CAD build for the part. Positions are in the model's coordinates, mm. A direction names the side the tool comes from. Give positions to 0.01 mm unless a question says otherwise; leave off trailing zeros. Loops run counter-clockwise (first coordinate to the right, second up) from the corner with the lowest first, then second, coordinate; pieces in that order, holes last. Notation, with made-up numbers: M 46.5,35.25 L 76.5,35.25 A22 cw 76.5,43.25 Z; hole C 71.5,73.25 d3. An arc over 180 degrees is marked long. Answer as CSV lines item,"result".
from build123d import *

# Parameters (mm, degrees)
F0_W     = 177.8
F0_H     = 177.8
F1_DEPTH = 12.7
F2_W     = 177.8
F2_H     = 177.8
F2_W_2   = 165.1
F2_H_2   = 165.1
F3_DEPTH = 50.8
F4_W     = 76.2
F4_H     = 25.4
F5_DEPTH = 177.8
F6_W     = 76.2
F6_H     = 25.4
F7_DEPTH = 177.8
F8_R     = 1.5875
F9_DEPTH = 25.4


with BuildPart() as f1:
    # F0 (on Top) → F1 (new body)
    with BuildSketch(Plane.XY):
        with Locations((88.9, 88.9)):
            Rectangle(F0_W, F0_H)
    extrude(amount=F1_DEPTH)

    # F2 (on face) → F3 (join)
    with BuildSketch(Plane.XY.offset(12.7)):
        with Locations((88.9, 88.9)):
            Rectangle(F2_W, F2_H)
        with Locations((88.9, 88.9)):
            Rectangle(F2_W_2, F2_H_2, mode=Mode.SUBTRACT)
    extrude(amount=F3_DEPTH)

    # F4 (on face) → F5 (cut, through all)
    with BuildSketch(Plane.YZ.offset(177.8)):
        with Locations((88.9, 38.1)):
            Rectangle(F4_W, F4_H)
    extrude(amount=-F5_DEPTH, mode=Mode.SUBTRACT)

    # F6 (on face) → F7 (cut, through all)
    with BuildSketch(Plane.XZ):
        with Locations((88.9, 38.1)):
            Rectangle(F6_W, F6_H)
    extrude(amount=-F7_DEPTH, mode=Mode.SUBTRACT)

    # F8 (on face) → F9 (join, through all)
    with BuildSketch(Plane.XY.offset(25.4)):
        with Locations((174.625, 69.85)):
            Circle(F8_R)
        with Locations((174.625, 57.15)):
            Circle(F8_R)
        with Locations((174.625, 82.55)):
            Circle(F8_R)
        with Locations((174.625, 107.95)):
            Circle(F8_R)
        with Locations((174.625, 120.65)):
            Circle(F8_R)
        with Locations((174.625, 95.25)):
            Circle(F8_R)
        with Locations((69.85, 174.625)):
            Circle(F8_R)
        with Locations((57.15, 174.625)):
            Circle(F8_R)
        with Locations((82.55, 174.625)):
            Circle(F8_R)
        with Locations((107.95, 174.625)):
            Circle(F8_R)
        with Locations((120.65, 174.625)):
            Circle(F8_R)
        with Locations((95.25, 174.625)):
            Circle(F8_R)
        with Locations((69.85, 3.175)):
            Circle(F8_R)
        with Locations((57.15, 3.175)):
            Circle(F8_R)
        with Locations((82.55, 3.175)):
            Circle(F8_R)
        with Locations((107.95, 3.175)):
            Circle(F8_R)
        with Locations((120.65, 3.175)):
            Circle(F8_R)
        with Locations((95.25, 3.175)):
            Circle(F8_R)
        with Locations((3.175, 69.85)):
            Circle(F8_R)
        with Locations((3.175, 57.15)):
            Circle(F8_R)
        with Locations((3.175, 82.55)):
            Circle(F8_R)
        with Locations((3.175, 107.95)):
            Circle(F8_R)
        with Locations((3.175, 120.65)):
            Circle(F8_R)
        with Locations((3.175, 95.25)):
            Circle(F8_R)
    extrude(amount=F9_DEPTH)


solid = f1.part
1) Which spindle directions (+Z, -Z, +X, -X, +Y, -Y) get a long thin tool onto all of the face, cutting with end or side? Do faces 5 (the face through (175, 127, 38)), 6 (the face through (50.8, 3, 38)), 7 (the face through (171.45, 88, 55)). Say none if no direction does.
Answer below:
face 5,"+X, -X"
face 6,"+Y, -Y"
face 7,"+Z"
2) Band-saw the part on C-C on z = 47. Give the number of separate pieces and of enclosed holes in the cut face, and give its area (3 significant figures).
Answer below:
separate pieces,"28"
enclosed holes,"0"
area,"2,610 mm^2"
3) Band-saw the part on A-A on x = 142.5. Give the cut face in (y, z), and give its area (3 significant figures).
Answer below:
outline,"M 0,0 L 177.8,0 L 177.8,63.5 L 171.45,63.5 L 171.45,12.7 L 6.35,12.7 L 6.35,63.5 L 0,63.5 Z"
area,"2,900 mm^2"
4) Mould opens along Z. For faces 1 (the face through (88, 90, 0)), 2 (the face through (88, 175, 25.4)), 3 (the face through (88, 6.35, 55)), 4 (the face through (88, 175, 50.8)) say: +Z half, -Z half, draft (parallel to the pull), parting line (faces both ways), or undercut.
Answer below:
face 1,"-Z half"
face 2,"undercut"
face 3,"draft"
face 4,"undercut"
5) Flat gauge pins, fed straight in: pin 1 (15 mm diameter, centred on y = 109, z = 36.5, fed in from +X); pin 2 (1 mm diameter, centred on y = 81.5, z = 47, fed in from -X); pin 3 (3 mm diameter, centred on x = 99.5, z = 30.5, fed in from +Y). Where does each tip first touch, or does it go through?
Answer below:
pin 1,"stops at x = 176.21"
pin 2,"stops at x = 1.69"
pin 3,"passes through"
6) Drill centre lines: line 1 (X direction, y = 98, z = 53.5); line 2 (X direction, y = 95, z = 33). Where is each one in solid material? Low to high. Write a range as from..to.
Answer below:
line 1,"x = 0..6.35, 171.45..177.8"
line 2,"x = 1.61..4.74, 173.06..176.19"
